Can you work these out from the model? Positions are in its coordinate system, mm. Face numbers are marked on the shaded views. A direction names the side the tool comes from. Round coordinates to 2 decimals unless told otherwise and drop trailing zeros. Write each loop counter-clockwise with the first axis right and the second up, starting at its lowest first coordinate (ties: lowest second). Pieces come first, ordered by that corner, then holes. Notation, with made-up numbers: M 5.25,-34 L 16.25,-34 A20 cw 16.25,-29 Z; hole C 5,44.25 d9. An arc over 180 degrees is marked long. Answer as a JSON object with one key per item and string values. Group by question number.
1) Please list where these lines run through material, in increasing order: L1, parallel to Z at x = 0, y = 17.5; L2, parallel to Z at x = -32.5, y = -0.5; L3, parallel to Y at x = 9.5, z = 60.5. Write a range as [from, to].
2) Suppose I cut it at C-C, the plane y = -20.5. Write out the boundary of the cut face in (x, z).
3) On a 3-axis mill with a long thin cutter (end or side, diameter ignored), from which of +Z, -Z, +X, -X, +Y, -Y can I reach the whole of each face in a straight line? I mean the marked faces 5, 6, 7, 8 and 9. Say none if no direction works.
4) Suppose I cut it at A-A, the plane x = 0. Write out the boundary of the cut face in (y, z).
5) Suppose I cut it at B-B, the plane z = 42.5. Write out the boundary of the cut face in (x, y).
6) Suppose I cut it at D-D, the plane y = 18. Write out the boundary of the cut face in (x, z) (3 decimals), and give its area (3 significant figures).
7) I'm going to push flat-ended pins straight in: pin 1 Ø13 at (y, z) = (14.5, 67) entering from -X; pin 2 Ø14 at (x, y) = (-0.5, -14.5) entering from +Z; pin 3 Ø3.5 at (y, z) = (13, 65.5) entering from +X. Where does each tip first touch, or does it pass through?
8) If we mould it in two halves opening along X, with no side actions, what happens to the marked faces 1, 2, 3 and 4? For each: +X half, -X half, draft (parallel to the pull), parting line (faces both ways), or undercut.
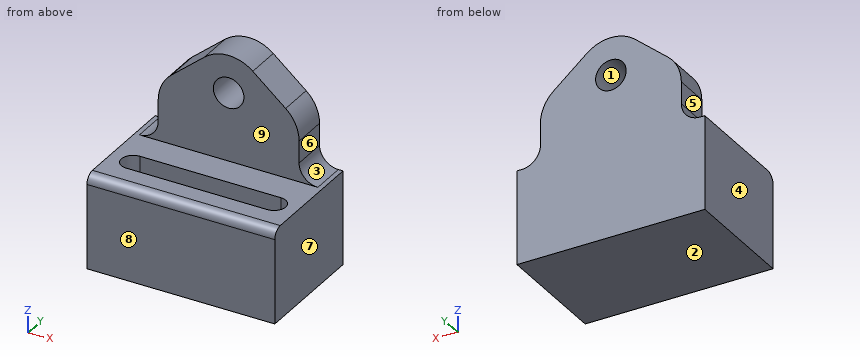
from build123d import *

# Parameters (mm, degrees)
F0_W      = 101.6
F0_H      = 63.5
F1_DEPTH  = 50.8
F2_R      = 5.08
F4_DEPTH  = 12.7
F5_W      = 101.6
F5_H      = 19.05
F6_DEPTH  = 63.5
F8_DEPTH  = 25.4
F9_R      = 20.32
F10_R     = 10.16
F11_R     = 8.255
F12_DEPTH = 25.4


with BuildPart() as f1:
    # F0 (on Top) → F1 (new body)
    with BuildSketch(Plane.XY):
        with Locations((0, -6.35)):
            Rectangle(F0_W, F0_H)
    extrude(amount=F1_DEPTH)

    # F2
    f2_edges = [f1.edges().sort_by_distance(p)[0] for p in [
        (0, -38.1, 50.8),
    ]]
    fillet(f2_edges, radius=F2_R)

    # F3 (on face) → F4 (cut)
    with BuildSketch(Plane.XY.offset(50.8)):
        with BuildLine():
            Line((38.1, -10.6305400074), (-38.1, -10.6305400074))
            ThreePointArc((-38.1, -10.6305400074), (-44.45, -16.9805400074), (-38.1, -23.3305400074))
            Line((-38.1, -23.3305400074), (38.1, -23.3305400074))
            ThreePointArc((38.1, -23.3305400074), (44.45, -16.9805400074), (38.1, -10.6305400074))
        make_face()
    extrude(amount=-F4_DEPTH, mode=Mode.SUBTRACT)

    # F5 (on face) → F6 (join)
    with BuildSketch(Plane.XY.offset(50.8)):
        with Locations((0, 15.875)):
            Rectangle(F5_W, F5_H)
    extrude(amount=F6_DEPTH)

    # F7 (on face) → F8 (cut)
    with BuildSketch(Plane.XZ.offset(-6.35)):
        Polygon((-50.8, 50.8), (-38.1, 50.8), (-38.1, 82.3303040521), (0, 114.3), (-50.8, 114.3), align=None)
        Polygon((38.1, 50.8), (50.8, 50.8), (50.8, 114.3), (0, 114.3), (38.1, 82.3303040521), align=None)
    extrude(amount=-F8_DEPTH, mode=Mode.SUBTRACT)

    # F9
    f9_edges = [f1.edges().sort_by_distance(p)[0] for p in [
        (38.1, 15.875, 82.330304),
        (-38.1, 15.875, 82.330304),
        (0, 15.875, 114.3),
    ]]
    fillet(f9_edges, radius=F9_R)

    # F10
    f10_edges = [f1.edges().sort_by_distance(p)[0] for p in [
        (38.1, 15.875, 50.8),
        (-38.1, 15.875, 50.8),
    ]]
    fillet(f10_edges, radius=F10_R)

    # F11 (on face) → F12 (cut)
    with BuildSketch(Plane.XZ.offset(-6.35)):
        with Locations((0, 87.7741238808)):
            Circle(F11_R)
    extrude(amount=-F12_DEPTH, mode=Mode.SUBTRACT)


solid = f1.part
Results:
{
 "1": {"L1": "[0, 79.52], [96.03, 108.09]", "L2": "[0, 50.8]", "L3": "[6.35, 25.4]"},
 "2": {"outline": "M -50.8,0 L 50.8,0 L 50.8,50.8 L 43.39,50.8 L 43.39,38.1 L -43.39,38.1 L -43.39,50.8 L -50.8,50.8 Z"},
 "3": {"face 5": "+Z, -X, +Y, -Y", "face 6": "+Z, +X, +Y, -Y", "face 7": "+Z, -Z, +X, +Y, -Y", "face 8": "+Z, -Z, +X, -X, -Y", "face 9": "+Z, +X, -X, -Y"},
 "4": {"outline": "M -38.1,0 L 25.4,0 L 25.4,79.52 L 6.35,79.52 L 6.35,50.8 L -10.63,50.8 L -10.63,38.1 L -23.33,38.1 L -23.33,50.8 L -33.02,50.8 A5.08 ccw -38.1,45.72 Z; M 6.35,96.03 L 25.4,96.03 L 25.4,108.09 L 6.35,108.09 Z"},
 "5": {"outline": "M -50.8,-38.1 L 50.8,-38.1 L 50.8,25.4 L -50.8,25.4 Z; hole M -38.1,-23.33 L 38.1,-23.33 A6.35 ccw 38.1,-10.63 L -38.1,-10.63 A6.35 ccw Z"},
 "6": {"outline": "M -50.8,0 L 50.8,0 L 50.8,50.8 L 48.26,50.8 A10.16 cw 38.1,60.96 L 38.1,72.855 A20.32 ccw 30.841,88.421 L 13.061,103.34 A20.32 ccw -13.061,103.34 L -30.841,88.421 A20.32 ccw -38.1,72.855 L -38.1,60.96 A10.16 cw -48.26,50.8 L -50.8,50.8 Z; hole C 0,87.774 d16.51", "area": "8,530 mm^2"},
 "7": {"pin 1": "x = -38.11", "pin 2": "z = 50.8", "pin 3": "x = 38.1"},
 "8": {"face 1": "undercut", "face 2": "draft", "face 3": "+X half", "face 4": "-X half"}
}
